from build123d import *

# Parameters (mm, degrees)
F1_DEPTH = 152.4
F2_DEPTH = 25.4
F3_DEPTH = 101.6
F0_R     = 57.15
F4_DEPTH = 127


with BuildPart() as f1:
    # F0 (on Front) → F1 (new body)
    with BuildSketch(Plane.XZ):
        Polygon((101.599478, -203.715121), (101.599478, -152.915121), (12.7, -152.73483), (-12.7, -152.683317), (-152.4, -152.4), (-152.4, -203.2), align=None)
    extrude(amount=F1_DEPTH)

    # F0 (on Front) → F2 (join)
    with BuildSketch(Plane.XZ):
        with BuildLine():
            ThreePointArc((75.245546, 12.022802), (75.961012, 6.030314), (76.2, 0))
            ThreePointArc((76.2, 0), (58.198711, -49.186888), (12.7, -75.134213))
            Line((12.7, -75.134213), (12.7, -152.73483))
            Line((12.7, -152.73483), (101.599478, -152.915121))
            Line((101.599478, -152.915121), (75.245546, 12.022802))
        make_face()
        with BuildLine():
            ThreePointArc((-12.7, -75.134213), (-67.246003, -35.838737), (-69.451562, 31.351562))
            Line((-69.451562, 31.351562), (-152.4, -152.4))
            Line((-152.4, -152.4), (-12.7, -152.683317))
            Line((-12.7, -152.683317), (-12.7, -152.4))
            Line((-12.7, -152.4), (-12.7, -75.134213))
        make_face()
    extrude(amount=F2_DEPTH)

    # F0 (on Front) → F3 (join)
    with BuildSketch(Plane.XZ):
        with BuildLine():
            Line((12.7, -152.73483), (12.7, -75.134213))
            ThreePointArc((12.7, -75.134213), (0, -76.2), (-12.7, -75.134213))
            Line((-12.7, -75.134213), (-12.7, -152.4))
            Line((-12.7, -152.4), (-12.7, -152.683317))
            Line((-12.7, -152.683317), (12.7, -152.73483))
        make_face()
    extrude(amount=F3_DEPTH)

    # F0 (on Front) → F4 (join)
    with BuildSketch(Plane.XZ):
        with BuildLine():
            ThreePointArc((12.7, -75.134213), (58.198711, -49.186888), (76.2, 0))
            ThreePointArc((76.2, 0), (75.961012, 6.030314), (75.245546, 12.022802))
            ThreePointArc((75.245546, 12.022802), (10.089242, 75.529115), (-69.451562, 31.351562))
            ThreePointArc((-69.451562, 31.351562), (-67.246003, -35.838737), (-12.7, -75.134213))
            ThreePointArc((-12.7, -75.134213), (0, -76.2), (12.7, -75.134213))
        make_face()
        Circle(F0_R, mode=Mode.SUBTRACT)
    extrude(amount=F4_DEPTH)


solid = f1.part
Source: CAD feature listing. Evaluate the final solid. Frame: model axes, mm. A direction names the side the tool comes from. Round coordinates to 2 decimals unless told otherwise and drop trailing zeros. Loops run counter-clockwise (first coordinate to the right, second up) from the corner with the lowest first, then second, coordinate; pieces in that order, holes last. Notation, with made-up numbers: M -29,-11.75 L 11,-11.75 A19 cw 11,11.25 Z; hole C -1.5,42.25 d7. An arc over 180 degrees is marked long. Return JSON: item names as keys, results as strings. Group by question number.
1. Mould query, pull axis X, two halves, no side actions, for faces 6 (the face through (-110.345, -12.522, -59.238)), 7 (the face through (-27, 0, -93)), 8 (the face through (-57.095, -62.611, 2.513)). Classes: released by +X, released by -X, zero draft, split by the parting line, or undercut.
2. Reachability of faces 1 (the face through (57, -25.4, -106)), 2 (the face through (-0.2, -114.1, -76.2)), 3 (the face through (75.968, -75.489, 5.946)), 4 (the face through (-68, -25.4, -100)), 5 (the face through (11, -127, 57)) from +Z, -Z, +X, -X, +Y, -Y: full face, straight path, thin tool, end or side. Return the list, or none.
3. Pin query (flat end, axial travel): pin 1 (8 mm diameter, centred on y = -41.5, z = -39.5, fed in from +X); pin 2 (4 mm diameter, centred on y = -37, z = 35, fed in from +X); pin 3 (12 mm diameter, centred on x = -69.5, y = -31, fed in from +Z); pin 4 (3 mm diameter, centred on x = -106.5, z = -93.5, fed in from +Y). Return the tip coordinate at first contact, or that it passes through.
4. Section query A-A on x = 0. Output: boundary loops of the cut face in (y, z), and give its area (3 significant figures).
5. Section query B-B on y = -42. Output: boundary loops of the cut face in (x, z).
6. Section query D-D on y = -135. Output: boundary loops of the cut face in (x, z).
7. Section query C-C on z = 41. Output: boundary loops of the cut face in (x, y).
8. Material intervals for line 1 along Z through (x, y) = (-27, -32.5); line 2 along X through (y, z) = (-53, -88); line 3 along Z through (x, y) = (85.5, -78), sorted ascending. Write a range as from..to.
Checks:
{
 "1": {"face 6": "released by -X", "face 7": "zero draft", "face 8": "undercut"},
 "2": {"face 1": "+X, -Y", "face 2": "-Y", "face 3": "+Z, +X, -Y", "face 4": "-X, -Y", "face 5": "+Z, +X, -X, -Y"},
 "3": {"pin 1": "stops at x = 67.43", "pin 2": "stops at x = 68.68", "pin 3": "stops at z = 42.12", "pin 4": "stops at y = 0"},
 "4": {"outline": "M -152.4,-203.51 L 0,-203.51 L 0,-57.15 L -127,-57.15 L -127,-76.2 L -101.6,-76.2 L -101.6,-152.71 L -152.4,-152.71 Z; M -127,57.15 L 0,57.15 L 0,76.2 L -127,76.2 Z", "area": "20,400 mm²"},
 "5": {"outline": "M -152.4,-203.2 L 101.6,-203.72 L 101.6,-152.92 L 12.7,-152.73 L 12.7,-75.13 A76.2 ccw 76.2,0 A76.2 ccw 75.25,12.02 A76.2 ccw -69.45,31.35 A76.2 ccw -12.7,-75.13 L -12.7,-152.68 L -152.4,-152.4 Z; hole C 0,0 d114.3"},
 "6": {"outline": "M -152.4,-203.2 L 101.6,-203.72 L 101.6,-152.92 L -152.4,-152.4 Z"},
 "7": {"outline": "M -64.23,-127 L -39.81,-127 L -39.81,0 L -64.23,0 Z; M 39.81,-127 L 64.23,-127 L 64.23,0 L 39.81,0 Z"},
 "8": {"line 1": "z = -203.45..-152.65, -71.26..-50.37, 50.37..71.26", "line 2": "x = -12.7..12.7", "line 3": "z = -203.68..-152.88"}
}
